from build123d import *

# Parameters (mm, degrees)
SKETCH_1_W      = 145
SKETCH_1_H      = 130
SKETCH_1_R      = 2.25
EXTRUDE_1_DEPTH = 1.5


with BuildPart() as part:
    # Эскиз1 → Вытянуть1 (new body)
    with BuildSketch(Plane.XY):
        Rectangle(SKETCH_1_W, SKETCH_1_H)
        with Locations((-67.5, 60)):
            Circle(SKETCH_1_R, mode=Mode.SUBTRACT)
        with Locations(Location((-67.5, -60, 0), (0, 0, 180))):
            Circle(SKETCH_1_R, mode=Mode.SUBTRACT)
        with Locations((67.5, -60)):
            Circle(SKETCH_1_R, mode=Mode.SUBTRACT)
        with Locations(Location((67.5, 60, 0), (0, 0, 180))):
            Circle(SKETCH_1_R, mode=Mode.SUBTRACT)
        with Locations((-67.5, 45)):
            Circle(SKETCH_1_R, mode=Mode.SUBTRACT)
        with Locations(Location((-67.5, -45, 0), (0, 0, 180))):
            Circle(SKETCH_1_R, mode=Mode.SUBTRACT)
        with Locations((62.5, 45)):
            Circle(SKETCH_1_R, mode=Mode.SUBTRACT)
        with Locations(Location((62.5, -45, 0), (0, 0, 180))):
            Circle(SKETCH_1_R, mode=Mode.SUBTRACT)
    extrude(amount=EXTRUDE_1_DEPTH)


solid = part.part
Can you work these out from the model? Positions are in its coordinate system, mm. Give positions to 0.01 mm unless a question says otherwise; leave off trailing zeros. Loops run counter-clockwise (first coordinate to the right, second up) from the corner with the lowest first, then second, coordinate; pieces in that order, holes last. Notation, with made-up numbers: M 72.25,42.25 L 92.25,42.25 A27 ccw 92.25,77.25 Z; hole C 74,54.5 d10. An arc over 180 degrees is marked long. One line per item, written item: value.
1) Please list where these lines run through material, in increasing order: line 1 (X direction, y = -45, z = 1.05); line 2 (Y direction, x = -67.5, z = 0.55); line 3 (Y direction, x = 62.5, z = 1).
Geometry check:
line 1: x = -72.5 to -69.75, -65.25 to 60.25, 64.75 to 72.5
line 2: y = -65 to -62.25, -57.75 to -47.25, -42.75 to 42.75, 47.25 to 57.75, 62.25 to 65
line 3: y = -65 to -47.25, -42.75 to 42.75, 47.25 to 65
2) Imagine slicing it at A-A on y = -60. Write out the boundary of the cut face in (x, z).
Geometry check:
outline: M -72.5,0 L -69.75,0 L -69.75,1.5 L -72.5,1.5 Z; M -65.25,0 L 65.25,0 L 65.25,1.5 L -65.25,1.5 Z; M 69.75,0 L 72.5,0 L 72.5,1.5 L 69.75,1.5 Z
3) I'm going to push a flat-ended pin straight in: pin 1 (4 mm diameter, centred on x = -67.5, y = -60, fed in from +Z). Where does the tip first touch, or does it pass through?
Geometry check:
pin 1: passes through
4) Imagine slicing it at B-B on x = -67.5. Write out the boundary of the cut face in (y, z).
Geometry check:
outline: M -65,0 L -62.25,0 L -62.25,1.5 L -65,1.5 Z; M -57.75,0 L -47.25,0 L -47.25,1.5 L -57.75,1.5 Z; M -42.75,0 L 42.75,0 L 42.75,1.5 L -42.75,1.5 Z; M 47.25,0 L 57.75,0 L 57.75,1.5 L 47.25,1.5 Z; M 62.25,0 L 65,0 L 65,1.5 L 62.25,1.5 Z
5) Thinking about a two-plate mould opening in Y: for faces 1 (the face through (-1, 1, 1.5)), 2 (the face through (64.16, -46.52, 0.74)), which applies, +Y half, -Y half, draft (parallel to the pull), parting line (faces both ways), or undercut?
Geometry check:
face 1: draft
face 2: undercut
6) Imagine slicing it at C-C on x = 67.5. Write out the boundary of the cut face in (y, z).
Geometry check:
outline: M -65,0 L -62.25,0 L -62.25,1.5 L -65,1.5 Z; M -57.75,0 L 57.75,0 L 57.75,1.5 L -57.75,1.5 Z; M 62.25,0 L 65,0 L 65,1.5 L 62.25,1.5 Z
